```python
from build123d import *

# Parameters (mm, degrees)
BOSS_EXTRUDE1_DEPTH      = 10
BOSS_EXTRUDE1_DEPTH_BACK = 10
SKETCH1_R                = 27.5
BOSS_EXTRUDE2_DEPTH      = 12
BOSS_EXTRUDE2_DEPTH_BACK = 12
SKETCH1_3_R              = 100
SKETCH1_3_R_2            = 85
BOSS_EXTRUDE3_DEPTH      = 5
BOSS_EXTRUDE3_DEPTH_BACK = 5
SKETCH1_4_R              = 85
SKETCH1_4_R_2            = 27.5
SKETCH2_R                = 7
CUT_EXTRUDE1_DEPTH       = 144.122325303
SKETCH3_R                = 3
SKETCH3_R_2              = 8
CUT_EXTRUDE2_DEPTH       = 144.122325303
SKETCH4_R                = 25
CUT_EXTRUDE3_DEPTH       = 143.439460825
CIRPATTERN1_COUNT        = 6


with BuildPart() as part:
    # Sketch1 → Boss-Extrude1 (new, two sides: drawn at the far end of the back side and taken through both)
    with BuildSketch(Plane.XY.offset(-BOSS_EXTRUDE1_DEPTH_BACK)):
        Circle(SKETCH1_R)
    extrude(amount=BOSS_EXTRUDE1_DEPTH + BOSS_EXTRUDE1_DEPTH_BACK)



with BuildPart() as body_2:
    # Sketch1_3 → Boss-Extrude2 (new, two sides: drawn at the far end of the back side and taken through both)
    with BuildSketch(Plane.XY.offset(-BOSS_EXTRUDE2_DEPTH_BACK)):
        Circle(SKETCH1_3_R)
        Circle(SKETCH1_3_R_2, mode=Mode.SUBTRACT)
    extrude(amount=BOSS_EXTRUDE2_DEPTH + BOSS_EXTRUDE2_DEPTH_BACK)


with BuildPart() as part_1:
    add(part.part)

    add(body_2.part)  # Boss-Extrude3 merges body 2
    # Sketch1_4 → Boss-Extrude3 (add, two sides: drawn at the far end of the back side and taken through both)
    with BuildSketch(Plane.XY.offset(-BOSS_EXTRUDE3_DEPTH_BACK)):
        Circle(SKETCH1_4_R)
        Circle(SKETCH1_4_R_2, mode=Mode.SUBTRACT)
    extrude(amount=BOSS_EXTRUDE3_DEPTH + BOSS_EXTRUDE3_DEPTH_BACK)

    # Sketch2 → Cut-Extrude1 (cut, through all)
    with BuildSketch(Plane.XY.offset(10)):
        Circle(SKETCH2_R)
    extrude(amount=-CUT_EXTRUDE1_DEPTH, mode=Mode.SUBTRACT)

    # Sketch3 → Cut-Extrude2 (cut, through all)
    with BuildSketch(Plane.XY.offset(10)):
        with Locations((0, 22)):
            Circle(SKETCH3_R)
        with Locations((0, 72)):
            Circle(SKETCH3_R_2)
        with Locations((62.353829072, 36)):
            Circle(SKETCH3_R_2)
        with Locations((19.052558883, 11)):
            Circle(SKETCH3_R)
        with Locations((62.353829072, -36)):
            Circle(SKETCH3_R_2)
        with Locations((19.052558883, -11)):
            Circle(SKETCH3_R)
        with Locations((0, -72)):
            Circle(SKETCH3_R_2)
        with Locations((0, -22)):
            Circle(SKETCH3_R)
        with Locations((-62.353829072, -36)):
            Circle(SKETCH3_R_2)
        with Locations((-19.052558883, -11)):
            Circle(SKETCH3_R)
        with Locations((-62.353829072, 36)):
            Circle(SKETCH3_R_2)
        with Locations((-19.052558883, 11)):
            Circle(SKETCH3_R)
    extrude(amount=-CUT_EXTRUDE2_DEPTH, mode=Mode.SUBTRACT)

    # Sketch4 → Cut-Extrude3 (cut, through all)
    with BuildSketch(Plane(origin=(0, 0, -5), x_dir=(-1, 0, 0), z_dir=(0, 0, -1))):
        with Locations((27.851651468, 47.426632924)):
            Circle(SKETCH4_R)
    cut_extrude3 = extrude(amount=-CUT_EXTRUDE3_DEPTH, mode=Mode.SUBTRACT)

    # CirPattern1: Cut-Extrude3 ×6 about axis
    cirpattern1_axis = Axis((0, 0, 0), (0, 0, 1))
    for i in range(1, CIRPATTERN1_COUNT):
        add(cut_extrude3.rotate(cirpattern1_axis, i * 360 / CIRPATTERN1_COUNT), mode=Mode.SUBTRACT)


solid = part_1.part
```
The model under review builds one solid part; all positions refer to its coordinate system, in mm. A direction names the side the tool comes from. Coordinates: 2 decimals unless noted, no trailing zeros. Write each loop counter-clockwise with the first axis right and the second up, starting at its lowest first coordinate (ties: lowest second). Pieces come first, ordered by that corner, then holes.
1) Machinability: for faces 1 (the face through (-67.453, -51.721, 8.451)), 2 (the face through (56.46, 41.41, 0.07)), 3 (the face through (-67.453, -51.721, -8.549)), which of the approach directions +Z, -Z, +X, -X, +Y, -Y give a long, thin tool a straight path to every point of the face, cutting with its end or side? Answer none if there is none.
2) We need section C-C on y = -36. State the section outline as (x, z) points, then the cut area to 3 significant figures.
3) Clearance check with flat-ended pins moving along their axes: pin 1 Ø2 at (x, z) = (41.5, -9.5) entering from +Y; pin 2 Ø18 at (x, y) = (0, 0) entering from -Z; pin 3 Ø13 at (x, y) = (62.35, 36) entering from -Z; pin 4 Ø3 at (y, z) = (51.5, -0.5) entering from +X. State where each tip first meets the part, or that it passes through.
4) To check wall thickness, follow probe 1 along Y at (x, z) = (0, 4.25); probe 2 along Y at (x, z) = (-43.5, 3.75); probe 3 along X at (y, z) = (54, -3.5). State the ranges of each line that lie inside material, in increasing order.
5) The part is to be moulded in two halves that separate along Y. For faces 4 (the face through (-45, -74, 12)), 5 (the face through (7.31, 63.05, -0.07)), 6 (the face through (95.38, 30.04, -0.17)), say which applies: pulls with the +Y half, pulls with the -Y half, needs draft (parallel to the pull), parting line crosses it, or undercut.
6) We need section B-B on x = 40. State the section outline as (y, z) points.
7) We need section A-A on y = -56.5. State the section outline as (x, z) points.
8) We need section D-D on x = -59. State the section outline as (y, z) points, then the cut area to 3 significant figures.
Answer list:
1. face 1: +Z
1. face 2: +Z, -Z
1. face 3: -Z
2. outline: (-93.3, -12) - (-77, -12) - (-77, -5) - (-70.35, -5) - (-70.35, 5) - (-77, 5) - (-77, 12) - (-93.3, 12) - close; (-54.35, -5) - (-49.17, -5) - (-49.17, 5) - (-54.35, 5) - close; (-5.12, -5) - (5.62, -5) - (5.62, 5) - (-5.12, 5) - close; (50.09, -5) - (54.35, -5) - (54.35, 5) - (50.09, 5) - close; (70.35, -5) - (77, -5) - (77, -12) - (93.3, -12) - (93.3, 12) - (77, 12) - (77, 5) - (70.35, 5) - close
2. area: 1,120 mm2
3. pin 1: stops at y = 91.43
3. pin 2: stops at z = -10
3. pin 3: passes through
3. pin 4: stops at x = 86.6
4. probe 1: y = -100 to -80, -64 to -25, -19 to -7, 7 to 19, 25 to 64, 80 to 100
4. probe 2: y = -90.04 to -66.74, -28.92 to -22.61, 21.79 to 27.93, 66.92 to 90.04
4. probe 3: x = -84.17 to -51.97, -3.73 to 2.92, 51.37 to 84.17
5. face 4: needs draft
5. face 5: undercut
5. face 6: parting line crosses it
6. outline: (-91.65, -12) - (-75, -12) - (-75, -5) - (-69.28, -5) - (-69.28, 5) - (-75, 5) - (-75, 12) - (-91.65, 12) - close; (-25.58, -5) - (-19.59, -5) - (-19.59, 5) - (-25.58, 5) - close; (20.41, -5) - (26.39, -5) - (26.39, 5) - (20.41, 5) - close; (69.28, -5) - (75, -5) - (75, -12) - (91.65, -12) - (91.65, 12) - (75, 12) - (75, 5) - (69.28, 5) - close
7. outline: (-82.51, -12) - (-63.5, -12) - (-63.5, -5) - (-50.6, -5) - (-50.6, 5) - (-63.5, 5) - (-63.5, 12) - (-82.51, 12) - close; (-3.7, -5) - (4.56, -5) - (4.56, 5) - (-3.7, 5) - close; (51.15, -5) - (63.5, -5) - (63.5, -12) - (82.51, -12) - (82.51, 12) - (63.5, 12) - (63.5, 5) - (51.15, 5) - close
8. outline: (-80.74, -12) - (-61.19, -12) - (-61.19, -5) - (-43.26, -5) - (-43.26, 5) - (-61.19, 5) - (-61.19, 12) - (-80.74, 12) - close; (-28.74, -5) - (-25.08, -5) - (-25.08, 5) - (-28.74, 5) - close; (24.27, -5) - (28.74, -5) - (28.74, 5) - (24.27, 5) - close; (43.26, -5) - (61.19, -5) - (61.19, -12) - (80.74, -12) - (80.74, 12) - (61.19, 12) - (61.19, 5) - (43.26, 5) - close
8. area: 1,380 mm2
